from build123d import *

# Parameters (mm, degrees)
SKETCH1_W                = 64
SKETCH1_H                = 304
SKETCH1_R                = 3
BOSS_EXTRUDE1_DEPTH      = 1
EDGE_FLANGE1_DEPTH       = 304
EDGE_FLANGE1_START       = 1
EDGE_FLANGE1_PROFILE_R   = 7.5
EDGE_FLANGE1_PROFILE_R_2 = 20
EDGE_FLANGE1_FLAT_DEPTH  = 1
EDGE_FLANGE2_DEPTH       = 260
EDGE_FLANGE2_START       = -1
EDGE_FLANGE2_PROFILE_R   = 3
EDGE_FLANGE2_FLAT_DEPTH  = 1
EDGE_FLANGE3_DEPTH       = 87
EDGE_FLANGE3_START       = -1
EDGE_FLANGE3_PROFILE_R   = 3
EDGE_FLANGE3_FLAT_DEPTH  = 1
EDGE_FLANGE4_DEPTH       = 304
EDGE_FLANGE4_START       = 1
EDGE_FLANGE4_PROFILE_W   = 304
EDGE_FLANGE4_PROFILE_H   = 43.5
EDGE_FLANGE4_PROFILE_R   = 4
EDGE_FLANGE4_FLAT_DEPTH  = 1
EDGE_FLANGE5_DEPTH       = 43.5
EDGE_FLANGE5_START       = 1
EDGE_FLANGE5_PROFILE_R   = 3
EDGE_FLANGE5_FLAT_DEPTH  = 1


# Sheet-metal steps are written as plain solids
with BuildPart() as part:
    # Sketch1 → Boss-Extrude1 (new body)
    with BuildSketch(Plane.XY):
        Rectangle(SKETCH1_W, SKETCH1_H)
        Circle(SKETCH1_R, mode=Mode.SUBTRACT)
        with Locations((0, 76)):
            Circle(SKETCH1_R, mode=Mode.SUBTRACT)
        with Locations((0, -76)):
            Circle(SKETCH1_R, mode=Mode.SUBTRACT)
    extrude(amount=BOSS_EXTRUDE1_DEPTH)

    # Edge-Flange1 bend section (across the edge) → Edge-Flange1 (add)
    with BuildSketch(Plane(origin=(-34, 152, 1), x_dir=(1, 0, 0), z_dir=(0, -1, 0))):
        with BuildLine():
            Line((-1, 2), (0, 2))
            ThreePointArc((0, 2), (0.585786438, 0.585786438), (2, 0))
            Line((2, 0), (2, -1))
            ThreePointArc((2, -1), (-0.121320344, -0.121320344), (-1, 2))
        make_face()
    extrude(amount=EDGE_FLANGE1_DEPTH)

    # Edge-Flange1 profile (on flange) → Edge-Flange1 flat (add)
    with BuildSketch(Plane(origin=(-34, 0, 1), x_dir=(0, -1, 0), z_dir=(-1, 0, 0)).offset(EDGE_FLANGE1_START)):
        with BuildLine():
            ThreePointArc((152, 89), (130, 87), (108, 89))
            Line((108, 89), (-152, 89))
            Line((-152, 89), (-152, 2))
            Line((-152, 2), (152, 2))
            Line((152, 2), (152, 89))
        make_face()
        with Locations((-132, 44.5)):
            Circle(EDGE_FLANGE1_PROFILE_R, mode=Mode.SUBTRACT)
        with Locations((0, 44.5)):
            Circle(EDGE_FLANGE1_PROFILE_R_2, mode=Mode.SUBTRACT)
        with Locations((-132, 66.75)):
            Circle(EDGE_FLANGE1_PROFILE_R, mode=Mode.SUBTRACT)
    extrude(amount=-EDGE_FLANGE1_FLAT_DEPTH)

    # Edge-Flange2 bend section (across the edge) → Edge-Flange2 (add)
    with BuildSketch(Plane(origin=(-35, -108, 92), x_dir=(0, 0, -1), z_dir=(0, 1, 0))):
        with BuildLine():
            Line((-1, 2), (0, 2))
            ThreePointArc((0, 2), (0.585786438, 0.585786438), (2, 0))
            Line((2, 0), (2, -1))
            ThreePointArc((2, -1), (-0.121320344, -0.121320344), (-1, 2))
        make_face()
    extrude(amount=EDGE_FLANGE2_DEPTH)

    # Edge-Flange2 profile (on flange) → Edge-Flange2 flat (add)
    with BuildSketch(Plane(origin=(-35, 0, 92), x_dir=(0, -1, 0), z_dir=(0, 0, -1)).offset(EDGE_FLANGE2_START)):
        with BuildLine():
            Line((-152, 2), (108, 2))
            Line((108, 2), (108, 18))
            ThreePointArc((108, 18), (107.414213562, 19.414213562), (106, 20))
            Line((106, 20), (-150, 20))
            ThreePointArc((-150, 20), (-151.414213562, 19.414213562), (-152, 18))
            Line((-152, 18), (-152, 2))
        make_face()
        with Locations((43, 10)):
            Circle(EDGE_FLANGE2_PROFILE_R, mode=Mode.SUBTRACT)
        with Locations((-87, 10)):
            Circle(EDGE_FLANGE2_PROFILE_R, mode=Mode.SUBTRACT)
    extrude(amount=EDGE_FLANGE2_FLAT_DEPTH)

    # Edge-Flange3 bend section (across the edge) → Edge-Flange3 (add)
    with BuildSketch(Plane(origin=(-35, 154, 90), x_dir=(0, -1, 0), z_dir=(0, 0, -1))):
        with BuildLine():
            Line((-1, 2), (0, 2))
            ThreePointArc((0, 2), (0.585786438, 0.585786438), (2, 0))
            Line((2, 0), (2, -1))
            ThreePointArc((2, -1), (-0.121320344, -0.121320344), (-1, 2))
        make_face()
    edge_flange3 = extrude(amount=EDGE_FLANGE3_DEPTH)

    # Edge-Flange3 profile (on flange) → Edge-Flange3 flat (add)
    with BuildSketch(Plane(origin=(-35, 154, 0), x_dir=(0, 0, 1), z_dir=(0, -1, 0)).offset(EDGE_FLANGE3_START)):
        with BuildLine():
            Line((3, 2), (90, 2))
            Line((90, 2), (90, 18))
            ThreePointArc((90, 18), (89.414213562, 19.414213562), (88, 20))
            Line((88, 20), (5, 20))
            ThreePointArc((5, 20), (3.585786438, 19.414213562), (3, 18))
            Line((3, 18), (3, 2))
        make_face()
        with Locations((24.75, 10)):
            Circle(EDGE_FLANGE3_PROFILE_R, mode=Mode.SUBTRACT)
        with Locations((68.25, 10)):
            Circle(EDGE_FLANGE3_PROFILE_R, mode=Mode.SUBTRACT)
    edge_flange3_flat = extrude(amount=EDGE_FLANGE3_FLAT_DEPTH)

    # Mirror1: Edge-Flange3, Edge-Flange3 flat across plane
    add(edge_flange3.mirror(Plane.ZX))
    add(edge_flange3_flat.mirror(Plane.ZX))

    # Edge-Flange4 bend section (across the edge) → Edge-Flange4 (add)
    with BuildSketch(Plane(origin=(34, -152, 1), x_dir=(-1, 0, 0), z_dir=(0, 1, 0))):
        with BuildLine():
            Line((-1, 2), (0, 2))
            ThreePointArc((0, 2), (0.585786438, 0.585786438), (2, 0))
            Line((2, 0), (2, -1))
            ThreePointArc((2, -1), (-0.121320344, -0.121320344), (-1, 2))
        make_face()
    extrude(amount=EDGE_FLANGE4_DEPTH)

    # Edge-Flange4 profile (on flange) → Edge-Flange4 flat (add)
    with BuildSketch(Plane(origin=(34, 0, 1), x_dir=(0, 1, 0), z_dir=(1, 0, 0)).offset(EDGE_FLANGE4_START)):
        with Locations((0, 23.75)):
            Rectangle(EDGE_FLANGE4_PROFILE_W, EDGE_FLANGE4_PROFILE_H)
        with Locations((-76, 22.75)):
            Circle(EDGE_FLANGE4_PROFILE_R, mode=Mode.SUBTRACT)
        with Locations((76, 22.75)):
            Circle(EDGE_FLANGE4_PROFILE_R, mode=Mode.SUBTRACT)
    extrude(amount=-EDGE_FLANGE4_FLAT_DEPTH)

    # Edge-Flange5 bend section (across the edge) → Edge-Flange5 (add)
    with BuildSketch(Plane(origin=(35, 154, 3), x_dir=(0, -1, 0), z_dir=(0, 0, 1))):
        with BuildLine():
            Line((-1, 2), (0, 2))
            ThreePointArc((0, 2), (0.585786438, 0.585786438), (2, 0))
            Line((2, 0), (2, -1))
            ThreePointArc((2, -1), (-0.121320344, -0.121320344), (-1, 2))
        make_face()
    edge_flange5 = extrude(amount=EDGE_FLANGE5_DEPTH)

    # Edge-Flange5 profile (on flange) → Edge-Flange5 flat (add)
    with BuildSketch(Plane(origin=(35, 154, 0), x_dir=(0, 0, 1), z_dir=(0, 1, 0)).offset(EDGE_FLANGE5_START)):
        with BuildLine():
            ThreePointArc((5, 20), (3.585786438, 19.414213562), (3, 18))
            Line((3, 18), (3, 2))
            Line((3, 2), (46.5, 2))
            Line((46.5, 2), (46.5, 18))
            ThreePointArc((46.5, 18), (45.914213562, 19.414213562), (44.5, 20))
            Line((44.5, 20), (5, 20))
        make_face()
        with Locations((24.75, 10)):
            Circle(EDGE_FLANGE5_PROFILE_R, mode=Mode.SUBTRACT)
    edge_flange5_flat = extrude(amount=-EDGE_FLANGE5_FLAT_DEPTH)

    # Mirror2: Edge-Flange5, Edge-Flange5 flat across plane
    add(edge_flange5.mirror(Plane.ZX))
    add(edge_flange5_flat.mirror(Plane.ZX))


solid = part.part
Build history of the part. All positions in model axes, mm. A direction names the side the tool comes from. Coordinates: 2 decimals unless noted, no trailing zeros. Order: outer loops, then holes, each group sorted by start corner. A loop starts at its lowest first (then second) coordinate and runs counter-clockwise, first axis right, second up. Notation, with made-up numbers: (-24.5, 43) - (9.5, 43) arc R23 ccw to (9.5, 75) - close; hole circle Ø7 at (-23.5, 57). An arc over 180 degrees is marked (long way). Write each question's results on one line, items separated by ' | '. Start each with the question number.
Item 1: Tool access for faces 1 (the face through (34.3, -0.7, 46.5)), 2 (the face through (-34, 2, 66)), 3 (the face through (-34.51, 2.6, 65.33)), 4 (the face through (-46, 24, 92)): list every direction of +Z, -Z, +X, -X, +Y, -Y with a clear straight run to the whole face (end or side of a thin tool).
Item 2: Mould opens along Z. For faces 5 (the face through (35, -2, 25)), 6 (the face through (-8, 2, 0)), 7 (the face through (-47.974, -154.507, 24.359)) say: released by +Z, released by -Z, zero draft, split by the parting line, or undercut.
Item 3: Wall check: probe 1 along Z at (x, y) = (-45, -154.6); probe 2 along Y at (x, z) = (0, 0.65); probe 3 along Y at (x, z) = (-47.5, 16.5). Give the ranges that are in metal, low to high. Write a range as [from, to].
Item 4: Band-saw the part on B-B on z = 11. Write the cut outline in (x, y), and give its area (3 significant figures).
Item 5: Band-saw the part on A-A on y = 132. Write the cut outline in (x, z).
Item 6: Flat gauge pins, fed straight in: pin 1 (4 mm diameter, centred on y = 77, z = 69.5, fed in from +X); pin 2 (12 mm diameter, centred on y = -24, z = 66, fed in from -X); pin 3 (0.9 mm diameter, centred on x = -11.5, z = 1, fed in from -Y). Where does each tip first touch, or does it go through?
Item 7: Band-saw the part on D-D on y = -76. Write the cut outline in (x, z).
Item 8: Band-saw the part on C-C on x = 45. Write the cut outline in (y, z).
Numbers:
1) face 1: +Z, +X, +Y, -Y | face 2: +Z, +Y, -Y | face 3: -X | face 4: -Z, -X, +Y, -Y
2) face 5: zero draft | face 6: released by -Z | face 7: undercut
3) probe 1: [3, 21.75], [27.75, 65.25], [71.25, 90] | probe 2: [-152, -79], [-73, -3], [3, 73], [79, 152] | probe 3: [-155, -154], [154, 155]
4) outline: (-55, -155) - (-37, -155) arc R3 ccw to (-34, -152) - (-34, 152) arc R3 ccw to (-37, 155) - (-55, 155) - (-55, 154) - (-37, 154) arc R2 cw to (-35, 152) - (-35, -152) arc R2 cw to (-37, -154) - (-55, -154) - close; (34, -152) arc R3 ccw to (37, -155) - (55, -155) - (55, -154) - (37, -154) arc R2 cw to (35, -152) - (35, 152) arc R2 cw to (37, 154) - (55, 154) - (55, 155) - (37, 155) arc R3 ccw to (34, 152) - close | area: 696 mm^2
5) outline: (-55, 92) - (-37, 92) arc R2 cw to (-35, 90) - (-35, 75.25) - (-34, 75.25) - (-34, 90) arc R3 ccw to (-37, 93) - (-55, 93) - close; (-35, 3) arc R3 ccw to (-32, 0) - (32, 0) arc R3 ccw to (35, 3) - (35, 46.5) - (34, 46.5) - (34, 3) arc R2 cw to (32, 1) - (-32, 1) arc R2 cw to (-34, 3) - (-34, 38) - (-35, 38) - close; (-35, 53) - (-34, 53) - (-34, 60.25) - (-35, 60.25) - close
6) pin 1: x = -34 | pin 2: x = -35 | pin 3: y = -152
7) outline: (-55, 92) - (-37, 92) arc R2 cw to (-35, 90) - (-35, 3) arc R3 ccw to (-32, 0) - (-3, 0) - (-3, 1) - (-32, 1) arc R2 cw to (-34, 3) - (-34, 90) arc R3 ccw to (-37, 93) - (-55, 93) - close; (3, 0) - (32, 0) arc R3 ccw to (35, 3) - (35, 19.75) - (34, 19.75) - (34, 3) arc R2 cw to (32, 1) - (3, 1) - close; (34, 27.75) - (35, 27.75) - (35, 46.5) - (34, 46.5) - close
8) outline: (-155, 3) - (-154, 3) - (-154, 21.75) - (-155, 21.75) - close; (-155, 27.75) - (-154, 27.75) - (-154, 46.5) - (-155, 46.5) - close; (154, 3) - (155, 3) - (155, 21.75) - (154, 21.75) - close; (154, 27.75) - (155, 27.75) - (155, 46.5) - (154, 46.5) - close
